Could you check a few things on this model? Use its own coordinates, in mm. Coordinates: 2 decimals unless noted, no trailing zeros. Order: outer loops, then holes, each group sorted by start corner. A loop starts at its lowest first (then second) coordinate and runs counter-clockwise, first axis right, second up. Notation, with made-up numbers: (63, 74) - (74, 74) arc R17 cw to (74, 85) - close; hole circle Ø9 at (49.25, 29.5). An arc over 180 degrees is marked (long way). Answer as CSV lines item,"result". Start each with the question number.
1. I want a section at A-A, the plane z = 159.5. List the corners of the cut face in (x, y) for me.
2. For pin 1 (1 mm diameter, centred on x = 22.5, z = 127.5, fed in from -Y); pin 2 (6 mm diameter, centred on x = 43, y = -2.5, fed in from +Z); pin 3 (0.7 mm diameter, centred on x = -14, z = 128, fed in from -Y), each with a flat end and sliding along its axis, tell me the tip position at first contact or that it passes through.
3. I need wall thicknesses on probe 1 along X at (y, z) = (-6, 56) (3 decimals); probe 2 along Y at (x, z) = (-2, 45.5); probe 3 along Y at (x, z) = (0, 26). Which ranges of each line are inside material? Lowest first, please.
from build123d import *

# Parameters (mm, degrees)
F3_DEPTH  = 177.8
F4_R      = 7.62
F5_DEPTH  = 19.05
F6_SIZE2  = 18.860161823
F6_SIZE   = 7.62
F4_R_2    = 5.715
F7_DEPTH  = 5.08
F8_R      = 5.07999
F9_R      = 6.35
F10_DEPTH = 50.8
F11_SCALE = 1.1422


# Not quite as in the source:
# - a fillet or chamfer is up to 0.001 mm smaller than in the source, because OpenCascade refuses the exact size


with BuildPart() as f1:
    # F0 (on Front) → F1 (revolve)
    with BuildSketch(Plane.XZ):
        with BuildLine():
            Line((-38.2711647941, 0), (0, 0))
            Line((0, 0), (0, 146.0500033258))
            Line((0, 146.0500033258), (0, 152.4))
            ThreePointArc((0, 152.4), (-33.2006597867, 137.6319951518), (-44.4655865431, 103.0852268133))
            add(Edge.make_bspline(
                [(-44.4655865431, 0), (-47.1114422222, 11.762074058), (-53.3469479224, 35.8297600734), (-37.8272166921, 76.0482431769), (-42.543614325, 94.8604386904), (-44.4655865431, 103.0852268133)],
                knots=[0, 0, 0, 0, 0.3424224234, 0.7066775859, 1, 1, 1, 1], degree=3))
            Line((-44.4655865431, 0), (-38.2711647941, 0))
        make_face()
    revolve(axis=Axis((0, 0, 76.2), (0, 0, 1)))

    # F2 (on Top) → F3 (cut)
    with BuildSketch(Plane.XY):
        Polygon((25.6092443837, -36.641700535), (-25.1907556163, -36.641700535), (-46.7807556163, -36.641700535), (-46.7807556163, -67.121700535), (42.1192443837, -67.121700535), (42.1192443837, -36.641700535), align=None)
    extrude(amount=F3_DEPTH, mode=Mode.SUBTRACT)

    # F4 (on face) → F5 (join)
    with BuildSketch(Plane.XZ.offset(36.641700535)):
        with Locations((0, 97.9992443837)):
            Circle(F4_R)
    extrude(amount=F5_DEPTH)

    # F6
    f6_edges = [f1.edges().sort_by_distance(p)[0] for p in [
        (-7.62, -55.691701, 97.999244),
    ]]
    f6_side = f1.faces().sort_by_distance((0, -55.691701, 97.999244))[0]
    chamfer(f6_edges, length=F6_SIZE, length2=F6_SIZE2, reference=f6_side)

    # F4 (on face) → F7 (join)
    with BuildSketch(Plane.XZ.offset(36.641700535)):
        with Locations((-12.7, 112.2232443837)):
            Circle(F4_R_2)
        with Locations((12.7, 112.2232443837)):
            Circle(F4_R_2)
    extrude(amount=F7_DEPTH)

    # F8 (radius 5.08 in the source; OpenCascade refuses exactly that, so slightly less here)
    f8_edges = [f1.edges().sort_by_distance(p)[0] for p in [
        (-18.415, -41.721701, 112.223244),
        (6.985, -41.721701, 112.223244),
    ]]
    fillet(f8_edges, radius=F8_R)

    # F9 (on face) → F10 (cut)
    with BuildSketch(Plane(origin=(0, 0, 0), x_dir=(1, 0, 0), z_dir=(0, 0, -1))):
        Circle(F9_R)
    extrude(amount=-F10_DEPTH, mode=Mode.SUBTRACT)


with BuildPart() as f1_1:
    # F11: moved
    add(f1.part.scale(F11_SCALE))


solid = f1_1.part
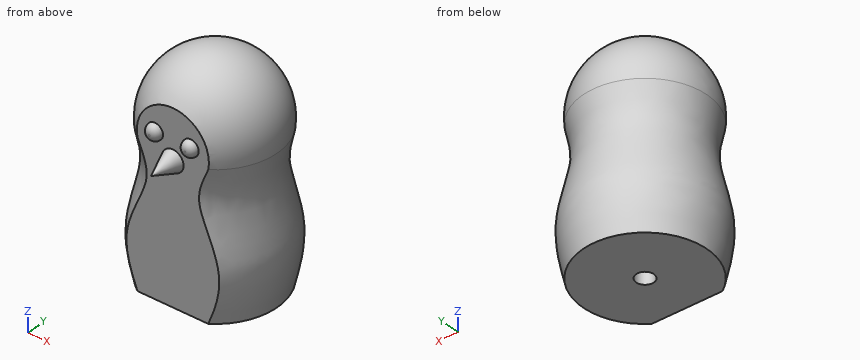
Solved:
1,outline,"circle Ø71.43 at (0, 0)"
2,pin 1,"stops at y = -41.85"
2,pin 2,"stops at z = 154.66"
2,pin 3,"stops at y = -47.65"
3,probe 1,"x = -53.384 to -4.075, 4.075 to 53.384"
3,probe 2,"y = -41.85 to -6.97, 6.97 to 55.6"
3,probe 3,"y = -41.85 to -7.25, 7.25 to 55.8"
